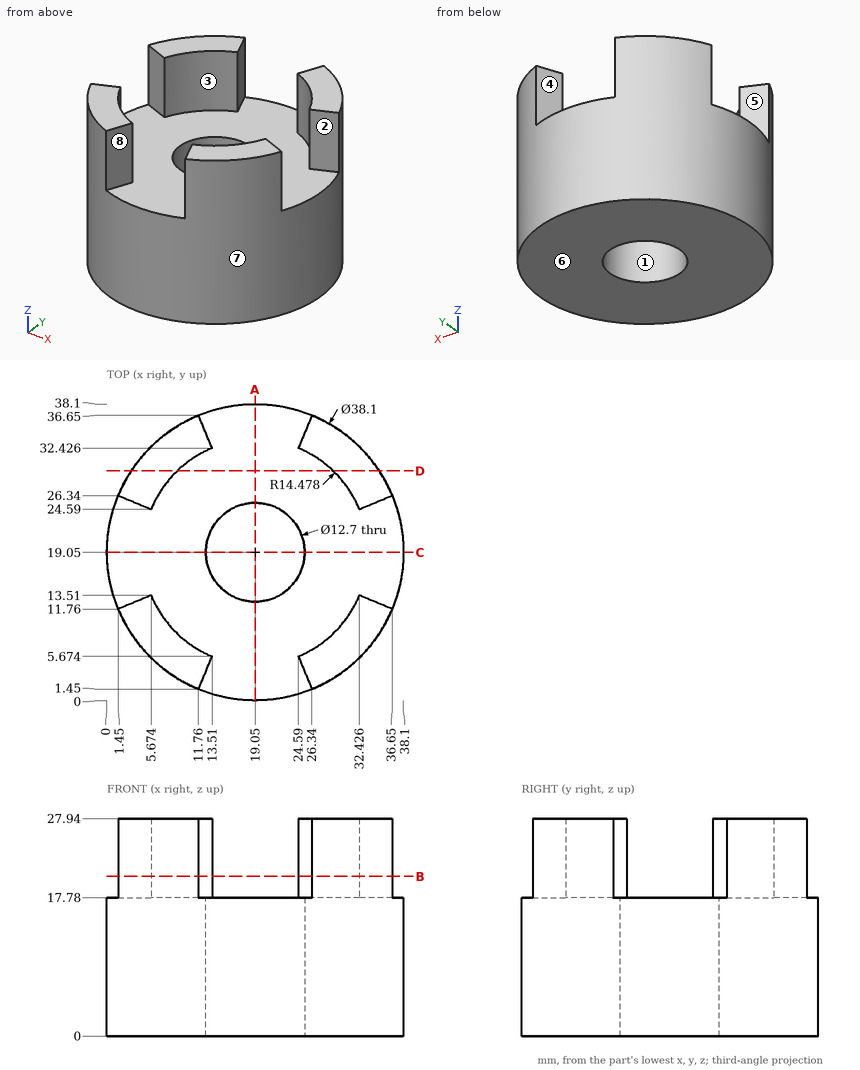
Source: three-view drawing plus pictorial views. Frame: mm from the lowest corner of the part. A direction names the side the tool comes from. Give positions to 0.01 mm unless a question says otherwise; leave off trailing zeros. Order: outer loops, then holes, each group sorted by start corner. A loop starts at its lowest first (then second) coordinate and runs counter-clockwise, first axis right, second up. Notation, with made-up numbers: M -26.75,-33.75 L 9.25,-33.75 A20 ccw 9.25,5.25 Z; hole C 47,8.25 d3. An arc over 180 degrees is marked long. Return JSON: item names as keys, results as strings.
1) Access query for the marked faces 1, 2, 3, 4 and 5. Directions: +Z, -Z, +X, -X, +Y, -Y. A direction counts if a zero-diameter tool reaches every point of the face in a straight line with its end or side. Return the directions, or none.
Taken from the geometry:
{"face 1": "+Z, -Z", "face 2": "+Z, +X", "face 3": "+Z", "face 4": "+Z, +Y", "face 5": "+Z, -X"}
2) Mould query, pull axis X, two halves, no side actions, for the marked faces 6, 7 and 8. Classes: released by +X, released by -X, zero draft, split by the parting line, or undercut.
Taken from the geometry:
{"face 6": "zero draft", "face 7": "split by the parting line", "face 8": "undercut"}
3) Section query B-B on z = 20.5. Count the separate pieces of the cut face and the enclosed holes in it, and give its area (3 significant figures).
Taken from the geometry:
{"separate pieces": "4", "enclosed holes": "0", "area": "241 mm2"}
4) Section query A-A on x = 19.05. Output: boundary loops of the cut face in (y, z).
Taken from the geometry:
{"outline": "M 0,0 L 12.7,0 L 12.7,17.78 L 0,17.78 Z; M 25.4,0 L 38.1,0 L 38.1,17.78 L 25.4,17.78 Z"}
5) Section query D-D on y = 29.5. Output: boundary loops of the cut face in (x, z).
Taken from the geometry:
{"outline": "M 3.12,0 L 34.98,0 L 34.98,27.94 L 29.07,27.94 L 29.07,17.78 L 9.03,17.78 L 9.03,27.94 L 3.12,27.94 Z"}
6) Line query: L1, parallel to Y at x = 19.05, z = 11; L2, parallel to Z at x = 16, y = 7; L3, parallel to X at y = 8.5, z = 21.25 (1 decimal). Output: solid intervals per line, ascending. Write a range as [from, to].
Taken from the geometry:
{"L1": "y = [0, 12.7], [25.4, 38.1]", "L2": "z = [0, 17.78]", "L3": "x = [3.2, 9.1], [29, 34.9]"}
7) Contact query for flat-ended pins moving along their axis: pin 1 (6 mm diameter, centred on x = 21, y = 31.5, fed in from +Z); pin 2 (8 mm diameter, centred on y = 10.5, z = 11, fed in from +X); pin 3 (1.5 mm diameter, centred on x = 13, z = 4.5, fed in from -Y). Output: stop coordinate, or through.
Taken from the geometry:
{"pin 1": "stops at z = 17.78", "pin 2": "stops at x = 37.55", "pin 3": "stops at y = 0.75"}
